Can you work these out from the model? Positions are in its coordinate system, mm. Face numbers are marked on the shaded views. Give positions to 0.01 mm unless a question says otherwise; leave off trailing zeros. Loops run counter-clockwise (first coordinate to the right, second up) from the corner with the lowest first, then second, coordinate; pieces in that order, holes last. Notation, with made-up numbers: (88, 41) - (117, 41) arc R23 ccw to (117, 51) - close; hole circle Ø9 at (80.5, 87.25). An arc over 180 degrees is marked (long way). Use a Markdown table: item, result. Add a question column.
```python
from build123d import *

# Parameters (mm, degrees)
F0_W     = 24
F0_H     = 14
F1_DEPTH = 20
F2_W     = 16
F2_H     = 8
F3_DEPTH = 18
F4_R     = 1.05
F5_DEPTH = 24.001


with BuildPart() as f1:
    # F0 (on Front) → F1 (new body)
    with BuildSketch(Plane.XZ):
        Rectangle(F0_W, F0_H)
    extrude(amount=F1_DEPTH)

    # F2 (on face) → F3 (cut)
    with BuildSketch(Plane(origin=(0, 0, 0), x_dir=(-1, 0, 0), z_dir=(0, 1, 0))):
        Rectangle(F2_W, F2_H)
    extrude(amount=-F3_DEPTH, mode=Mode.SUBTRACT)

    # F4 (on face) → F5 (cut, through all)
    with BuildSketch(Plane.YZ.offset(12)):
        with Locations((-15.35, 0)):
            Circle(F4_R)
        with Locations((-11.25, 0)):
            Circle(F4_R)
        with Locations((-3.05, 0)):
            Circle(F4_R)
        with Locations((-7.15, 0)):
            Circle(F4_R)
    extrude(amount=-F5_DEPTH, mode=Mode.SUBTRACT)


solid = f1.part
```
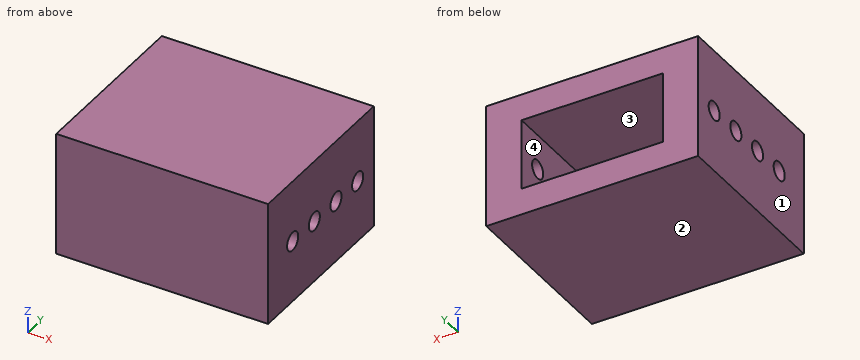
1. Suppose I cut it at B-B (x = -9.25). List the corners of the cut face in (y, z) for me, and give its area (3 significant figures).
2. If we mould it in two halves opening along Z, with no side actions, what happens to the marked faces 1, 2, 3 and 4? For each: released by +Z, released by -Z, zero draft, split by the parting line, or undercut.
3. Please list where these lines run through material, in increasing order: line 1 along Z through (x, y) = (-1.25, -9.5); line 2 along X through (y, z) = (-16.75, -1.5); line 3 along Z through (x, y) = (-10.65, -11.25). Write a range as [from, to].
4. Suppose I cut it at A-A (y = -11.25). List the corners of the cut face in (x, z) for me, and give its area (3 significant figures).
5. Will these pins go through, and if not, where does the flat tip stop? P1, Ø3.5, axis at y = -7.15, z = 0, coming from the +X side; P2, Ø1, axis at x = 3, z = 2.5, coming from the +Y side.
6. Suppose I cut it at D-D (z = 2). List the corners of the cut face in (x, y) for me, and give its area (3 significant figures).
7. Suppose I cut it at C-C (x = 4.75). List the corners of the cut face in (y, z) for me, and give its area (3 significant figures).
Results below:
| question | item | result |
|---|---|---|
| 1 | outline | (-20, -7) - (0, -7) - (0, 7) - (-20, 7) - close; hole circle Ø2.1 at (-15.35, 0); hole circle Ø2.1 at (-11.25, 0); hole circle Ø2.1 at (-7.15, 0); hole circle Ø2.1 at (-3.05, 0) |
| 1 | area | 266 mm² |
| 2 | face 1 | zero draft |
| 2 | face 2 | released by -Z |
| 2 | face 3 | undercut |
| 2 | face 4 | undercut |
| 3 | line 1 | [-7, -4], [4, 7] |
| 3 | line 2 | [-12, -8], [8, 12] |
| 3 | line 3 | [-7, -1.05], [1.05, 7] |
| 4 | outline | (-12, -7) - (12, -7) - (12, -1.05) - (8, -1.05) - (8, -4) - (-8, -4) - (-8, -1.05) - (-12, -1.05) - close; (-12, 1.05) - (-8, 1.05) - (-8, 4) - (8, 4) - (8, 1.05) - (12, 1.05) - (12, 7) - (-12, 7) - close |
| 4 | area | 191 mm² |
| 5 | P1 | x = 12 |
| 5 | P2 | y = -18 |
| 6 | outline | (-12, -20) - (12, -20) - (12, 0) - (8, 0) - (8, -18) - (-8, -18) - (-8, 0) - (-12, 0) - close |
| 6 | area | 192 mm² |
| 7 | outline | (-20, -7) - (0, -7) - (0, -4) - (-18, -4) - (-18, 4) - (0, 4) - (0, 7) - (-20, 7) - close |
| 7 | area | 136 mm² |
